from build123d import *

# Parameters (mm, degrees)
BOSS_EXTRUDE1_DEPTH = 10
BOSS_EXTRUDE2_DEPTH = 3
SKETCH3_R           = 10
BOSS_EXTRUDE3_DEPTH = 20
CUT_EXTRUDE1_DEPTH  = 11
CUT_EXTRUDE2_DEPTH  = 89


with BuildPart() as part:
    # Sketch1 → Boss-Extrude1 (new body)
    with BuildSketch(Plane(origin=(10, 0, 0), x_dir=(0, 0, -1), z_dir=(1, 0, 0))):
        with BuildLine():
            Line((0, 42.5), (-186, 42.5))
            ThreePointArc((-186, 42.5), (-228.5, 0), (-186, -42.5))
            Line((-186, -42.5), (0, -42.5))
            ThreePointArc((0, -42.5), (42.5, 0), (0, 42.5))
        make_face()
    extrude(amount=-BOSS_EXTRUDE1_DEPTH)

    # Sketch2 → Boss-Extrude2 (add)
    with BuildSketch(Plane.XZ.offset(42.5)):
        with BuildLine():
            Line((98.944350751, 17.892804965), (10, 0))
            Line((10, 0), (0, 0))
            Line((0, 0), (0, 186))
            Line((0, 186), (10, 186))
            Line((10, 186), (111.07737178, 49.396138729))
            ThreePointArc((111.07737178, 49.396138729), (113.663663971, 30.311978912), (98.944350751, 17.892804965))
        make_face()
    extrude(amount=BOSS_EXTRUDE2_DEPTH)

    # Sketch3 → Boss-Extrude3 (add)
    with BuildSketch(Plane.XZ.offset(45.5)):
        with Locations((95, 37.5)):
            Circle(SKETCH3_R)
    extrude(amount=BOSS_EXTRUDE3_DEPTH)

    # Sketch4 → Cut-Extrude1 (cut, through all)
    with BuildSketch(Plane(origin=(10, 0, 0), x_dir=(0, 0, -1), z_dir=(1, 0, 0))):
        with BuildLine():
            Line((-186, -20.390002673), (0, -20.390002673))
            ThreePointArc((0, -20.390002673), (20.390002673, 0), (0, 20.390002673))
            Line((0, 20.390002673), (-186, 20.390002673))
            ThreePointArc((-186, 20.390002673), (-206.390002673, 0), (-186, -20.390002673))
        make_face()
    extrude(amount=-CUT_EXTRUDE1_DEPTH, mode=Mode.SUBTRACT)

    # Sketch5 → Cut-Extrude2 (cut, through all)
    with BuildSketch(Plane.XZ.offset(45.5)):
        Polygon((13.715935026, 156.359237723), (13.715935026, 18.016014269), (64.102931729, 28.152292708), (80.693023557, 65.841164794), align=None)
    extrude(amount=-CUT_EXTRUDE2_DEPTH, mode=Mode.SUBTRACT)


solid = part.part
Design review of the part built by this model. Coordinates are the model's own, in mm. A direction names the side the tool comes from. Coordinates: 2 decimals unless noted, no trailing zeros. Order: outer loops, then holes, each group sorted by start corner. A loop starts at its lowest first (then second) coordinate and runs counter-clockwise, first axis right, second up. Notation, with made-up numbers: (-37.5, -39.5) - (-18.5, -39.5) arc R22 cw to (-18.5, -24.5) - close; hole circle Ø8 at (-8.75, -33). An arc over 180 degrees is marked (long way). Put each result on its own line as item: value.
1) Tool access review of faces 4 (the face through (5.07, -0.448, -20.385)), 5 (the face through (59.831, -43.979, 118.654)), 6 (the face through (10, 29, 95)), 7 (the face through (38.557, -44.021, 23.013)): name each direction out of +Z, -Z, +X, -X, +Y, -Y from which nothing blocks a thin tool from reaching the whole face with its end or side.
Response values:
face 4: +X, -X
face 5: +Z, +X, +Y, -Y
face 6: +Z, -Z, +X, +Y
face 7: +Y, -Y
2) Wall thickness on L1, parallel to Y at x = 12, z = 23; L2, parallel to X at y = -10.5, z = -30.5; L3, parallel to Y at x = 91, z = 31: over which ranges is each line inside the solid? List them lowest first. Write a range as from..to.
Response values:
L1: y = -45.5..-42.5
L2: x = 0..10
L3: y = -65.5..-42.5
3) The part is to be moulded in two halves that separate along X. For faces 1 (the face through (71, -45.5, 80)), 2 (the face through (72.28, -44.02, 46.73)), 3 (the face through (87.06, -55.36, 31.42)), say which applies: released by +X, released by -X, zero draft, split by the parting line, or undercut.
Response values:
face 1: zero draft
face 2: undercut
face 3: split by the parting line
4) Take a section at D-D, the plane z = 176.5. Give the boundary of the cut face in (x, y).
Response values:
outline: (0, -45.5) - (17.03, -45.5) - (17.03, -42.5) - (10, -42.5) - (10, -20.39) - (0, -20.39) - close; (0, 20.39) - (10, 20.39) - (10, 42.5) - (0, 42.5) - close
5) Take a section at A-A, the plane y = 0. Give the boundary of the cut face in (x, z).
Response values:
outline: (0, -42.5) - (10, -42.5) - (10, -20.39) - (0, -20.39) - close; (0, 206.39) - (10, 206.39) - (10, 228.5) - (0, 228.5) - close
6) Take a section at C-C, the plane x = 68. Give the boundary of the cut face in (y, z).
Response values:
outline: (-45.5, 11.67) - (-42.5, 11.67) - (-42.5, 37.01) - (-45.5, 37.01) - close; (-45.5, 83) - (-42.5, 83) - (-42.5, 107.61) - (-45.5, 107.61) - close
7) Insertion check: P1, Ø2.5, axis at y = -44.5, z = 73, coming from the +X side; P2, Ø12, axis at x = 90.5, y = -53, coming from the -Z side; P3, Ø2.5, axis at x = 6.5, y = -44, coming from the +Z side. Each pin has a flat end and moves straight along its axis. Give the tip position at first contact, or say it passes through.
Response values:
P1: stops at x = 94.54
P2: stops at z = 27.5
P3: stops at z = 186
8) Take a section at B-B, the plane z = 112. Give the boundary of the cut face in (x, y), and give its area (3 significant figures).
Response values:
outline: (0, -45.5) - (13.72, -45.5) - (13.72, -42.5) - (10, -42.5) - (10, -20.39) - (0, -20.39) - close; (0, 20.39) - (10, 20.39) - (10, 42.5) - (0, 42.5) - close; (46.54, -45.5) - (64.75, -45.5) - (64.75, -42.5) - (46.54, -42.5) - close
area: 538 mm²
